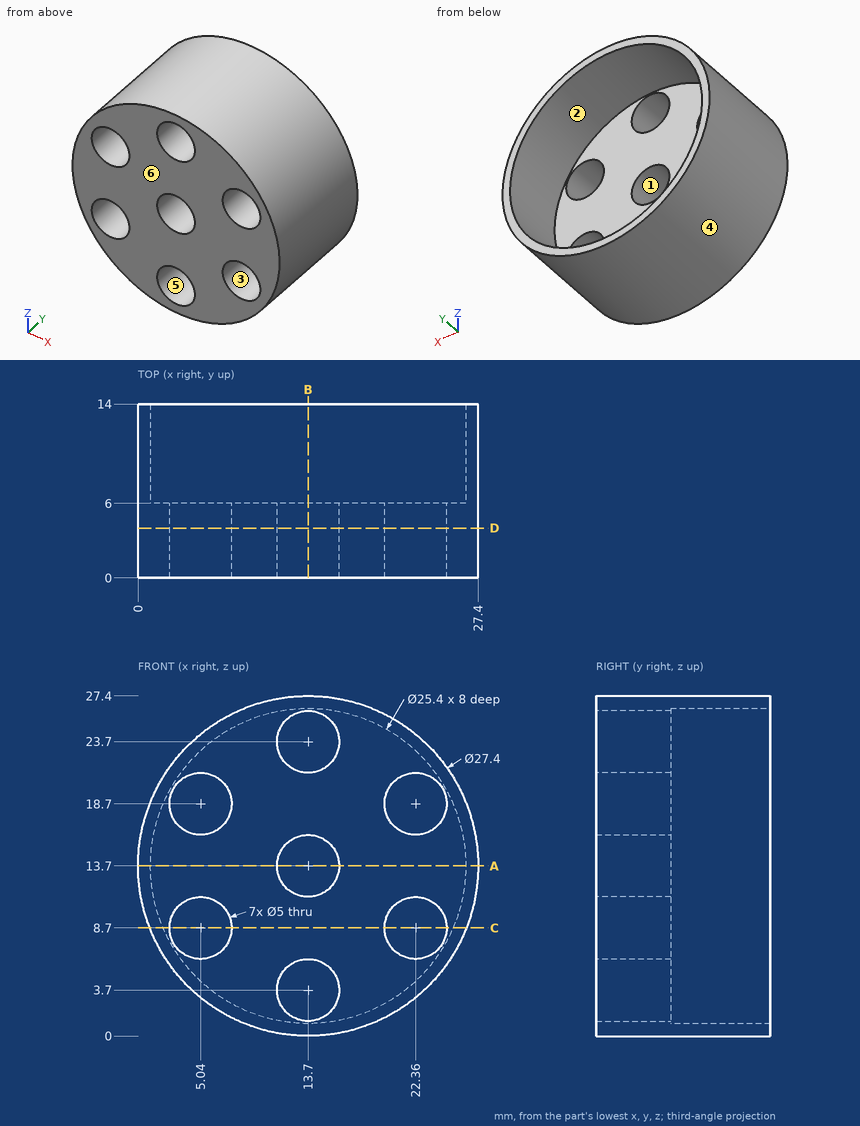
Verification items for this drawing (mm, ordinates from the low corner). A direction names the side the tool comes from. Round coordinates to 2 decimals unless told otherwise and drop trailing zeros. Loops run counter-clockwise (first coordinate to the right, second up) from the corner with the lowest first, then second, coordinate; pieces in that order, holes last. Notation, with made-up numbers: (35.5, -24) -> (60.5, -24) arc R20 ccw to (60.5, -9) -> close; hole circle Ø5 at (74.5, -36.5). An arc over 180 degrees is marked (long way). Answer in a Markdown table with one row per item.
Q1. Sectioned sample at B-B on x = 13.7. Enter the section's corners in (y, z).
Data:
| item | result |
|---|---|
| outline | (0, 0) -> (14, 0) -> (14, 1) -> (6, 1) -> (6, 1.2) -> (0, 1.2) -> close; (0, 6.2) -> (6, 6.2) -> (6, 11.2) -> (0, 11.2) -> close; (0, 16.2) -> (6, 16.2) -> (6, 21.2) -> (0, 21.2) -> close; (0, 26.2) -> (6, 26.2) -> (6, 26.4) -> (14, 26.4) -> (14, 27.4) -> (0, 27.4) -> close |
Q2. Sectioned sample at D-D on y = 4. Enter the section's corners in (x, z), then the cut area to 3 significant figures.
Data:
| item | result |
|---|---|
| outline | circle Ø27.4 at (13.7, 13.7); hole circle Ø5 at (5.04, 8.7); hole circle Ø5 at (5.04, 18.7); hole circle Ø5 at (13.7, 3.7); hole circle Ø5 at (13.7, 13.7); hole circle Ø5 at (13.7, 23.7); hole circle Ø5 at (22.36, 8.7); hole circle Ø5 at (22.36, 18.7) |
| area | 452 mm^2 |
Q3. Set-up check for the marked faces 1 and 2: record each of +Z, -Z, +X, -X, +Y, -Y from which the full face is reachable in a straight line by a thin tool's end or side.
Data:
| item | result |
|---|---|
| face 1 | +Y, -Y |
| face 2 | +Y |
Q4. Sectioned sample at A-A on z = 13.7. Enter the section's corners in (x, y).
Data:
| item | result |
|---|---|
| outline | (0, 0) -> (11.2, 0) -> (11.2, 6) -> (1, 6) -> (1, 14) -> (0, 14) -> close; (16.2, 0) -> (27.4, 0) -> (27.4, 14) -> (26.4, 14) -> (26.4, 6) -> (16.2, 6) -> close |
Q5. Thickness scan on L1, parallel to X at y = 2.05, z = 18.7 (1 decimal); L2, parallel to X at y = 2.15, z = 13.7; L3, parallel to Y at x = 7.25, z = 20. Record the ranges inside material, lowest first.
Data:
| item | result |
|---|---|
| L1 | x = 0.9 to 2.5, 7.5 to 19.9, 24.9 to 26.5 |
| L2 | x = 0 to 11.2, 16.2 to 27.4 |
| L3 | y = 0 to 6 |
Q6. Go/stop test with flat-tipped pins: P1, Ø2, axis at x = 20, z = 14.5, coming from the +Y side; P2, Ø5, axis at x = 24, y = 7, coming from the -Z side; P3, Ø8, axis at x = 5, y = 11, coming from the +Z side. Record where each tip stops, or that it passes through.
Data:
| item | result |
|---|---|
| P1 | stops at y = 6 |
| P2 | stops at z = 2.44 |
| P3 | stops at z = 26.57 |
Q7. Release check for a two-part mould opening along X. For the marked faces 3, 4, 5 and 6 record: released by +X, released by -X, zero draft, split by the parting line, or undercut.
Data:
| item | result |
|---|---|
| face 3 | undercut |
| face 4 | split by the parting line |
| face 5 | undercut |
| face 6 | zero draft |
Q8. Sectioned sample at C-C on z = 8.7. Enter the section's corners in (x, y) (1 decimal).
Data:
| item | result |
|---|---|
| outline | (0.9, 0) -> (2.5, 0) -> (2.5, 6) -> (2, 6) -> (2, 14) -> (0.9, 14) -> close; (7.5, 0) -> (19.9, 0) -> (19.9, 6) -> (7.5, 6) -> close; (24.9, 0) -> (26.5, 0) -> (26.5, 14) -> (25.4, 14) -> (25.4, 6) -> (24.9, 6) -> close |
